```python
from build123d import *

# Parameters (mm, degrees)
F0_W      = 26.555576
F0_H      = 26.555576
F0_R      = 9.525
F1_DEPTH  = 8.6995
F2_R      = 3.175
F3_R      = 11.1125
F4_DEPTH  = 7.112
F5_R      = 1.35255
F6_DEPTH  = 4.7625
F7_W      = 6.35
F7_H      = 6.35
F8_DEPTH  = 8.6995
F9_R      = 1.35255
F10_DEPTH = 4.7625


with BuildPart() as f1:
    # F0 (on Top) → F1 (new body)
    with BuildSketch(Plane.XY):
        Rectangle(F0_W, F0_H)
        Circle(F0_R, mode=Mode.SUBTRACT)
    extrude(amount=F1_DEPTH)

    # F2
    f2_edges = [f1.edges().sort_by_distance(p)[0] for p in [
        (-13.277788, 13.277788, 4.34975),
        (-13.277788, -13.277788, 4.34975),
        (13.277788, -13.277788, 4.34975),
        (13.277788, 13.277788, 4.34975),
    ]]
    fillet(f2_edges, radius=F2_R)

    # F3 (on face) → F4 (cut)
    with BuildSketch(Plane(origin=(0, 0, 0), x_dir=(1, 0, 0), z_dir=(0, 0, -1))):
        Circle(F3_R)
    extrude(amount=-F4_DEPTH, mode=Mode.SUBTRACT)

    # F5 (on face) → F6 (cut)
    with BuildSketch(Plane(origin=(0, 0, 0), x_dir=(1, 0, 0), z_dir=(0, 0, -1))):
        with Locations((10.102788, 10.102788)):
            Circle(F5_R)
        with Locations((-10.102788, 10.102788)):
            Circle(F5_R)
        with Locations((-10.102788, -10.102788)):
            Circle(F5_R)
        with Locations((10.102788, -10.102788)):
            Circle(F5_R)
    extrude(amount=-F6_DEPTH, mode=Mode.SUBTRACT)

    # F7 (on face) → F8 (join, through all)
    with BuildSketch(Plane.XY.offset(8.6995)):
        with Locations((4.7625, -16.452788)):
            Rectangle(F7_W, F7_H)
        with Locations((4.7625, 16.452788)):
            Rectangle(F7_W, F7_H)
    extrude(amount=-F8_DEPTH)

    # F9 (on face) → F10 (cut)
    with BuildSketch(Plane.YZ.offset(7.9375)):
        with Locations((16.452788, 3.175)):
            Circle(F9_R)
        with Locations((-16.452788, 3.175)):
            Circle(F9_R)
    extrude(amount=-F10_DEPTH, mode=Mode.SUBTRACT)


solid = f1.part
```
Geometry check sheet. Reference: the model listing, model coordinates, mm. A direction names the side the tool comes from. Coordinates: 2 decimals unless noted, no trailing zeros. Write each loop counter-clockwise with the first axis right and the second up, starting at its lowest first coordinate (ties: lowest second). Pieces come first, ordered by that corner, then holes. Notation, with made-up numbers: M 81,7 L 132,7 A11 ccw 132,25 Z; hole C 84.25,-40 d6. An arc over 180 degrees is marked long. One line per item, written item: value. Start each with the question number.
(1) Sectioned sample at D-D, the plane x = 5.5. Enter the section's corners in (y, z) (1 decimal).
(2) Depth check by flat-ended pin: pin 1 (2.5 mm diameter, centred on y = 16.45, z = 3.18, fed in from -X); pin 2 (0.8 mm diameter, centred on y = -16, z = 3.5, fed in from +X) (3 decimals); pin 3 (1.9 mm diameter, centred on y = 15.5, z = 5.5, fed in from +X). Enter the tip coordinate at first touch or a pass-through.
(3) Release check for a two-part mould opening along X. For faces 1 (the face through (3.175, -16, 3)), 2 (the face through (5.59, -15.163, 3.581)), 3 (the face through (10.6, -3.34, 3.51)) record: released by +X, released by -X, zero draft, split by the parting line, or undercut.
(4) Sectioned sample at A-A, the plane x = 0. Enter the section's corners in (y, z) (1 decimal).
(5) Scan lines: line 1 along Y through (x, z) = (-10, 3); line 2 along X through (y, z) = (0, 4.75); line 3 along X through (y, z) = (9, 4.5). Record each from-to range of solid material in increasing order. Write a range as [from, to].
(6) Tool access check on faces 4 (the face through (-4, 13.278, 4)), 5 (the face through (8.75, 10.04, 2.35)), 6 (the face through (7.938, -16, 5)), 7 (the face through (-4, -13.278, 4)). Record the directions out of +Z, -Z, +X, -X, +Y, -Y that give a thin tool (end or side, any length) a straight path to the whole face; none if there is none.
Filled sheet:
1. outline: M -19.6,0 L -9.7,0 L -9.7,7.1 L -7.8,7.1 L -7.8,8.7 L -19.6,8.7 Z; M 7.8,7.1 L 9.7,7.1 L 9.7,0 L 19.6,0 L 19.6,8.7 L 7.8,8.7 Z; hole C -16.5,3.2 d2.7; hole C 16.5,3.2 d2.7
2. pin 1: x = 1.59
2. pin 2: x = 3.175
2. pin 3: x = 7.94
3. face 1: released by +X
3. face 2: zero draft
3. face 3: undercut
4. outline: M -13.3,0 L -11.1,0 L -11.1,7.1 L -9.5,7.1 L -9.5,8.7 L -13.3,8.7 Z; M 9.5,7.1 L 11.1,7.1 L 11.1,0 L 13.3,0 L 13.3,8.7 L 9.5,8.7 Z
5. line 1: [-13.28, -11.45], [-8.75, -4.85], [4.85, 8.75], [11.45, 13.28]
5. line 2: [-13.28, -11.11], [11.11, 13.28]
5. line 3: [-13.28, -10.89], [-9.32, -6.52], [6.52, 9.32], [10.89, 13.28]
6. face 4: +Z, -Z, -X, +Y
6. face 5: -Z
6. face 6: +Z, -Z, +X, -Y
6. face 7: +Z, -Z, -X, -Y
